from build123d import *

# Parameters (mm, degrees)
SZKIC1_R                                    = 150
DODANIE_WYCI_GNI_CIE1_DEPTH                 = 6
OTWORY_USTALAJ_CE_8_0MM1_D                  = 8
OTWORY_USTALAJ_CE_8_0MM1_CSINK_D            = 8.05
OTWORY_USTALAJ_CE_8_0MM1_CSINK_ANGLE        = 90
POG_BIENIE_STO_KOWE_POD_M8_WKR_T_DO_2_COUNT = 2
POG_BIENIE_STO_KOWE_POD_M8_WKR_T_DO_2_PITCH = 190.91883092
POG_BIENIE_STO_KOWE_POD_M8_WKR_T_DO_3_COUNT = 2
POG_BIENIE_STO_KOWE_POD_M8_WKR_T_DO_3_PITCH = 270
POG_BIENIE_STO_KOWE_POD_M8_WKR_T_DO_4_COUNT = 2
POG_BIENIE_STO_KOWE_POD_M8_WKR_T_DO_4_PITCH = 190.91883092


with BuildPart() as part:
    # Szkic1 → Dodanie-wyciągnięcie1 (new body)
    with BuildSketch(Plane.XY):
        Circle(SZKIC1_R)
    extrude(amount=DODANIE_WYCI_GNI_CIE1_DEPTH)

    # Otwory ustalające Ø8.0mm1 (through all)
    with Locations(Plane.XY.offset(6)):
        with Locations((0, 70), (0, -70), (-70, 0), (70, 0)):
            CounterSinkHole(OTWORY_USTALAJ_CE_8_0MM1_D / 2, OTWORY_USTALAJ_CE_8_0MM1_CSINK_D / 2, counter_sink_angle=OTWORY_USTALAJ_CE_8_0MM1_CSINK_ANGLE)

    # Szkic6 → Otwory ustalające Ø12.0mm1 (revolve, cut)
    with BuildSketch(Plane(origin=(0, 0, 6), x_dir=(0, -1, 0), z_dir=(1, 0, 0))):
        Polygon((0, 0), (0, 6), (6, 6), (6, 0.025), (6.025, 0), align=None)
    revolve(axis=Axis((0, 0, 12.35), (0, 0, -1)), mode=Mode.SUBTRACT)

    # Szkic10 → Pogłębienie stożkowe pod M8 wkręt do części metalowych z łbem soczewkowym1 (revolve, cut)
    with BuildSketch(Plane(origin=(0, 135, 6), x_dir=(0, -1, 0), z_dir=(1, 0, 0))):
        Polygon((0, 0), (0, 6), (4.5, 6), (4.5, 4.15), (8.65, 0), align=None)
    pog_bienie_sto_kowe_pod_m8_wkr_t_do_cz_c = revolve(axis=Axis((0, 135, 12.35), (0, 0, -1)), mode=Mode.SUBTRACT)

    # Pog_bienie sto_kowe pod M8 wkr_t do  2: Pogłębienie stożkowe pod M8 wkręt do części metalowych z łbem soczewkowym1 ×2
    with Locations(*[Vector(0.7071067811865674, -0.7071067811865276, 0) * (i * POG_BIENIE_STO_KOWE_POD_M8_WKR_T_DO_2_PITCH) for i in range(1, POG_BIENIE_STO_KOWE_POD_M8_WKR_T_DO_2_COUNT)]):
        add(pog_bienie_sto_kowe_pod_m8_wkr_t_do_cz_c, mode=Mode.SUBTRACT)

    # Pog_bienie sto_kowe pod M8 wkr_t do  3: Pogłębienie stożkowe pod M8 wkręt do części metalowych z łbem soczewkowym1 ×2
    with Locations(*[(0, -i * POG_BIENIE_STO_KOWE_POD_M8_WKR_T_DO_3_PITCH, 0) for i in range(1, POG_BIENIE_STO_KOWE_POD_M8_WKR_T_DO_3_COUNT)]):
        add(pog_bienie_sto_kowe_pod_m8_wkr_t_do_cz_c, mode=Mode.SUBTRACT)

    # Pog_bienie sto_kowe pod M8 wkr_t do  4: Pogłębienie stożkowe pod M8 wkręt do części metalowych z łbem soczewkowym1 ×2
    with Locations(*[Vector(-0.7071067811865277, -0.7071067811865674, 0) * (i * POG_BIENIE_STO_KOWE_POD_M8_WKR_T_DO_4_PITCH) for i in range(1, POG_BIENIE_STO_KOWE_POD_M8_WKR_T_DO_4_COUNT)]):
        add(pog_bienie_sto_kowe_pod_m8_wkr_t_do_cz_c, mode=Mode.SUBTRACT)


solid = part.part
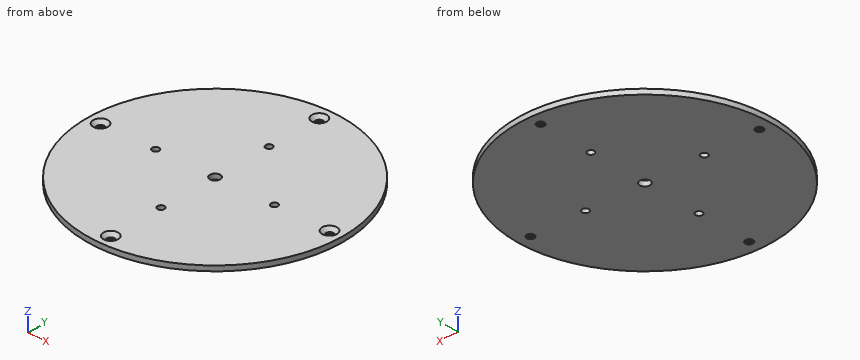
Model file for the job. Use its own axes, mm. Give positions to 0.01 mm unless a question says otherwise; leave off trailing zeros. Order: outer loops, then holes, each group sorted by start corner. A loop starts at its lowest first (then second) coordinate and runs counter-clockwise, first axis right, second up. Notation, with made-up numbers: (57, -21.75) - (64, -21.75) arc R23 ccw to (64, 9.25) - close; hole circle Ø2 at (20, 10.5). An arc over 180 degrees is marked (long way). Return JSON: item names as keys, results as strings.
1) Cut at A-A, the plane y = 0. Count the separate pieces of the cut face and the enclosed holes in it, plus the area to 3 significant figures.
Geometry says:
{"separate pieces": "6", "enclosed holes": "0", "area": "1,490 mm²"}
2) Probe line 1 (Y direction, x = 0, z = 1.6); line 2 (X direction, y = 6.5, z = 5.25); line 3 (Y direction, x = -0.5, z = 4). List the from-to ranges inside material, lowest first. Write a range as from..to.
Geometry says:
{"line 1": "-150..-139.5, -130.5..-74, -66..-6, 6..66, 74..130.5, 139.5..150", "line 2": "-149.86..-139.49, -130.51..130.51, 139.49..149.86", "line 3": "-150..-141.63, -128.37..-73.97, -66.03..-5.98, 5.98..66.03, 73.97..128.37, 141.63..150"}
3) Cut at D-D, the plane y = 70. Give the cut face in (x, z) (3 decimals), plus the area to 3 significant figures.
Geometry says:
{"outline": "(-132.665, 0) - (-4, 0) - (-4, 5.975) - (-4.025, 6) - (-132.665, 6) - close; (4, 0) - (132.665, 0) - (132.665, 6) - (4.025, 6) - (4, 5.975) - close", "area": "1,540 mm²"}
4) Cut at C-C, the plane x = 135. Give the cut face in (y, z).
Geometry says:
{"outline": "(-65.38, 0) - (-4.5, 0) - (-4.5, 1.85) - (-8.65, 6) - (-65.38, 6) - close; (4.5, 0) - (65.38, 0) - (65.38, 6) - (8.65, 6) - (4.5, 1.85) - close"}
5) Flat gauge pins, fed straight in: P1, Ø1.5, axis at x = -72, y = 120, coming from the -Z side; P2, Ø11.5, axis at x = 0, y = -135, coming from the +Z side; P3, Ø3, axis at y = 6.5, z = 5, coming from the +X side; P4, Ø1, axis at y = 96.5, z = 4.5, coming from the +X side. Where does each tip first touch, or does it go through?
Geometry says:
{"P1": "z = 0", "P2": "z = 3.1", "P3": "x = 149.92", "P4": "x = 115.26"}
